from build123d import *

# Parameters (mm, degrees)
SKETCH1_R                = 25
BOSS_EXTRUDE1_DEPTH      = 10
CHAMFER1_SIZE            = 5
CHAMFER1_SIZE2           = 2.886751346
CHAMFER2_SIZE            = 5
CHAMFER2_SIZE2           = 2.886751346
CUT_EXTRUDE1_DEPTH       = 37.742346142
CIRPATTERN1_COUNT        = 5
BOSS_EXTRUDE2_DEPTH      = 1
BOSS_EXTRUDE2_DEPTH_BACK = 12
SKETCH3_R                = 5


with BuildPart() as part:
    # Sketch1 → Boss-Extrude1 (new body)
    with BuildSketch(Plane.XY):
        Circle(SKETCH1_R)
    extrude(amount=BOSS_EXTRUDE1_DEPTH)

    # Chamfer1
    chamfer1_edges = [part.edges().sort_by_distance(p)[0] for p in [
        (-25, 0, 10),
    ]]
    chamfer1_side = [part.faces().sort_by_distance(p)[0] for p in [
        (0, 0, 10),
    ]]
    chamfer(chamfer1_edges, length=CHAMFER1_SIZE, length2=CHAMFER1_SIZE2, reference=chamfer1_side[0])

    # Chamfer2
    chamfer2_edges = [part.edges().sort_by_distance(p)[0] for p in [
        (-25, 0, 0),
    ]]
    chamfer2_side = [part.faces().sort_by_distance(p)[0] for p in [
        (0, 0, 0),
    ]]
    chamfer(chamfer2_edges, length=CHAMFER2_SIZE, length2=CHAMFER2_SIZE2, reference=chamfer2_side[0])

    # Sketch2 → Cut-Extrude1 (cut, through all)
    with BuildSketch(Plane.XY.offset(10)):
        with BuildLine():
            Line((11.23772214, 22.331896496), (4.095760221, 12.132117818))
            ThreePointArc((4.095760221, 12.132117818), (0, 10), (-4.095760221, 12.132117818))
            Line((-4.095760221, 12.132117818), (-11.23772214, 22.331896496))
            ThreePointArc((-11.23772214, 22.331896496), (0, 25), (11.23772214, 22.331896496))
        make_face()
    cut_extrude1 = extrude(amount=-CUT_EXTRUDE1_DEPTH, mode=Mode.SUBTRACT)

    # CirPattern1: Cut-Extrude1 ×5 about axis
    cirpattern1_axis = Axis((0, 0, 0), (0, 0, 1))
    for i in range(1, CIRPATTERN1_COUNT):
        add(cut_extrude1.rotate(cirpattern1_axis, i * 360 / CIRPATTERN1_COUNT), mode=Mode.SUBTRACT)

    # Sketch3 → Boss-Extrude2 (add, two sides: drawn at the far end of the back side and taken through both)
    with BuildSketch(Plane.XY.offset(10).offset(-BOSS_EXTRUDE2_DEPTH_BACK)):
        Circle(SKETCH3_R)
    extrude(amount=BOSS_EXTRUDE2_DEPTH + BOSS_EXTRUDE2_DEPTH_BACK)


solid = part.part
Verification items for the finished model (mm, model axes). A direction names the side the tool comes from. Give positions to 0.01 mm unless a question says otherwise; leave off trailing zeros. Write each loop counter-clockwise with the first axis right and the second up, starting at its lowest first coordinate (ties: lowest second). Pieces come first, ordered by that corner, then holes. Notation, with made-up numbers: M 47,51.5 L 73,51.5 A37 ccw 73,90.5 Z; hole C -13.75,19 d4. An arc over 180 degrees is marked long. Put each result on its own line as item: value. Start each with the question number.
1. Section check D-D (x = -6.5). Record the cut outline in (y, z).
2. Section check B-B (z = 5.5). Record the cut outline in (x, y), and give its area (3 significant figures).
3. Go/stop test with flat-tipped pins: pin 1 Ø2 at (y, z) = (-13.5, 2) entering from -X; pin 2 Ø5 at (y, z) = (16.5, 8) entering from +X; pin 3 Ø3 at (x, y) = (-6.5, 12.5) entering from -Z. Record where each tip stops, or that it passes through.
4. Draft check along X on faces 5 (the face through (-0.06, -22.53, 1.46)), 6 (the face through (-16.41, -9.46, 5.07)), 7 (the face through (0, 10, 5)), 8 (the face through (21.41, -7.02, 8.54)). Enter one of: +X half, -X half, draft (parallel to the pull), parting line (faces both ways), or undercut.
5. Section check A-A (x = 0). Record the cut outline in (y, z), and give its area (3 significant figures).
6. Section check C-C (z = 1.5). Record the cut outline in (x, y), and give its area (3 significant figures).
7. Scan lines: line 1 along Z through (x, y) = (-4, -8.5); line 2 along Y through (x, z) = (10, 6.5); line 3 along Y through (x, z) = (13.5, 1.75). Record each from-to range of solid material in increasing order. Write a range as [from, to].
8. Set-up check for faces 1 (the face through (4, 4, 0)), 2 (the face through (5.824, -8.13, 5.07)), 3 (the face through (4, 4, 10)), 4 (the face through (-18.67, -1.94, 5.07)): record each of +Z, -Z, +X, -X, +Y, -Y from which the full face is reachable in a straight line by a thin tool's end or side.
Answer list:
1. outline: M -7.7,0 L 15.57,0 L 15.57,10 L -7.7,10 Z
2. outline: M -24.71,-3.79 A25 ccw -22.22,-11.46 L -10.44,-7.41 A5 cw -3.82,-12.22 L -4.03,-24.67 A25 ccw 4.03,-24.67 L 3.82,-12.22 A5 cw 10.44,-7.41 L 22.22,-11.46 A25 ccw 24.71,-3.79 L 12.8,-0.15 A5 cw 10.27,7.64 L 17.77,17.59 A25 ccw 11.24,22.33 L 4.1,12.13 A5 cw -4.1,12.13 L -11.24,22.33 A25 ccw -17.77,17.59 L -10.27,7.64 A5 cw -12.8,-0.15 Z
2. area: 918 mm2
3. pin 1: x = -3.86
3. pin 2: x = 17.77
3. pin 3: z = 0
4. face 5: parting line
4. face 6: undercut
4. face 7: undercut
4. face 8: +X half
5. outline: M -25,2.89 L -20,0 L -5,0 L -5,-2 L 5,-2 L 5,0 L 10,0 L 10,10 L 5,10 L 5,11 L -5,11 L -5,10 L -20,10 L -25,7.11 Z
5. area: 366 mm2
6. outline: M -22.39,-3.08 A22.6 ccw -19.92,-10.67 L -10.44,-7.41 A5 cw -3.82,-12.22 L -3.99,-22.24 A22.6 ccw 3.99,-22.24 L 3.82,-12.22 A5 cw 10.44,-7.41 L 19.92,-10.67 A22.6 ccw 22.39,-3.08 L 12.8,-0.15 A5 cw 10.27,7.64 L 16.3,15.65 A22.6 ccw 9.84,20.34 L 4.1,12.13 A5 cw -4.1,12.13 L -9.84,20.34 A22.6 ccw -16.3,15.65 L -10.27,7.64 A5 cw -12.8,-0.15 Z
6. area: 821 mm2
7. line 1: [0, 10]
7. line 2: [-7.28, 2.03], [7.24, 20.56]
7. line 3: [-8.46, -0.36], [11.93, 18.66]
8. face 1: -Z
8. face 2: +Z, -Z
8. face 3: +Z
8. face 4: +Z, -Z, -X
